```python
from build123d import *

# Parameters (mm, degrees)
SKETCH1_W           = 20
SKETCH1_H           = 300
BOSS_EXTRUDE1_DEPTH = 15
SKETCH3_R           = 5
CUT_EXTRUDE1_DEPTH  = 15


with BuildPart() as part:
    # Sketch1 → Boss-Extrude1 (new body)
    with BuildSketch(Plane.XY):
        Rectangle(SKETCH1_W, SKETCH1_H)
    extrude(amount=BOSS_EXTRUDE1_DEPTH)

    # Sketch3 → Cut-Extrude1 (cut)
    with BuildSketch(Plane(origin=(0, 0, 0), x_dir=(-1, 0, 0), z_dir=(0, 0, -1))):
        with Locations((0, -140)):
            Circle(SKETCH3_R)
        with Locations((0, 140)):
            Circle(SKETCH3_R)
        with Locations((0, 60)):
            Circle(SKETCH3_R)
    extrude(amount=-CUT_EXTRUDE1_DEPTH, mode=Mode.SUBTRACT)


solid = part.part
```
Geometry: final body of the model. Coordinates: model frame, mm. Round coordinates to 2 decimals unless told otherwise and drop trailing zeros. Order: outer loops, then holes, each group sorted by start corner. A loop starts at its lowest first (then second) coordinate and runs counter-clockwise, first axis right, second up. Notation, with made-up numbers: (44, -19) -> (76, -19) arc R7 ccw to (76, -13) -> close; hole circle Ø8 at (67, 16.5). An arc over 180 degrees is marked (long way). Write each question's results on one line, items separated by ' | '.
Q1. Pull-direction query (Y, two-part tool) for faces 1 (the face through (-10, -2, 7)), 2 (the face through (0, -150, 7)), 3 (the face through (-2.307, -144.436, 7.395)), 4 (the face through (-3, 64, 7)); classes: released by +Y, released by -Y, zero draft, split by the parting line, or undercut.
Response values:
face 1: zero draft | face 2: released by -Y | face 3: undercut | face 4: undercut
Q2. Section query A-A (x = 0). Output: boundary loops of the cut face in (y, z), and give its area (3 significant figures).
Response values:
outline: (-150, 0) -> (-145, 0) -> (-145, 15) -> (-150, 15) -> close; (-135, 0) -> (55, 0) -> (55, 15) -> (-135, 15) -> close; (65, 0) -> (135, 0) -> (135, 15) -> (65, 15) -> close; (145, 0) -> (150, 0) -> (150, 15) -> (145, 15) -> close | area: 4,050 mm²
Q3. Section query C-C (z = 4.25). Output: boundary loops of the cut face in (x, y), and give its area (3 significant figures).
Response values:
outline: (-10, -150) -> (10, -150) -> (10, 150) -> (-10, 150) -> close; hole circle Ø10 at (0, -140); hole circle Ø10 at (0, 60); hole circle Ø10 at (0, 140) | area: 5,760 mm²
Q4. Pin query (flat end, axial travel): pin 1 Ø3 at (x, y) = (5.5, 28) entering from -Z; pin 2 Ø9 at (x, y) = (0, 140) entering from -Z. Return the tip coordinate at first contact, or that it passes through.
Response values:
pin 1: z = 0 | pin 2: through
Q5. Ray query, line 1 along Y through (x, z) = (0, 6.5); line 2 along Y through (x, z) = (3, 10). Return the intervals inside material, ascending.
Response values:
line 1: -150 to -145, -135 to 55, 65 to 135, 145 to 150 | line 2: -150 to -144, -136 to 56, 64 to 136, 144 to 150
Q6. Section query B-B (y = 60). Output: boundary loops of the cut face in (x, z).
Response values:
outline: (-10, 0) -> (-5, 0) -> (-5, 15) -> (-10, 15) -> close; (5, 0) -> (10, 0) -> (10, 15) -> (5, 15) -> close
